Here's the drawing with two shaded views (mm, measured from the low corner). I have some questions. Coordinates: 2 decimals unless noted, no trailing zeros. Order: outer loops, then holes, each group sorted by start corner. A loop starts at its lowest first (then second) coordinate and runs counter-clockwise, first axis right, second up. Notation, with made-up numbers: (-25.5, 30) -> (24.5, 30) arc R22 ccw to (24.5, 37) -> close; hole circle Ø7 at (14, 53). An arc over 180 degrees is marked (long way). Answer in a Markdown table with one row per item. Add a question column.
1. Imagine slicing it at B-B on x = 63. Write out the boundary of the cut face in (y, z), plus the area to 3 significant figures.
2. Will these pins go through, and if not, where does the flat tip stop? pin 1 (1.5 mm diameter, centred on x = 64.5, z = 1.5, fed in from +Y); pin 2 (1 mm diameter, centred on x = 17, z = 2.5, fed in from -Y).
3. Imagine slicing it at A-A on z = 1.8. Write out the boundary of the cut face in (x, y).
4. If I drill on line 1 along X through (y, z) = (50.5, 1.9); line 2 along Y through (x, z) = (39, 1.3), over which ranges is the centre line in solid material (lowest first)? Write a range as [from, to].
5. Imagine slicing it at C-C on x = 16.05. Write out the boundary of the cut face in (y, z), plus the area to 3 significant figures.
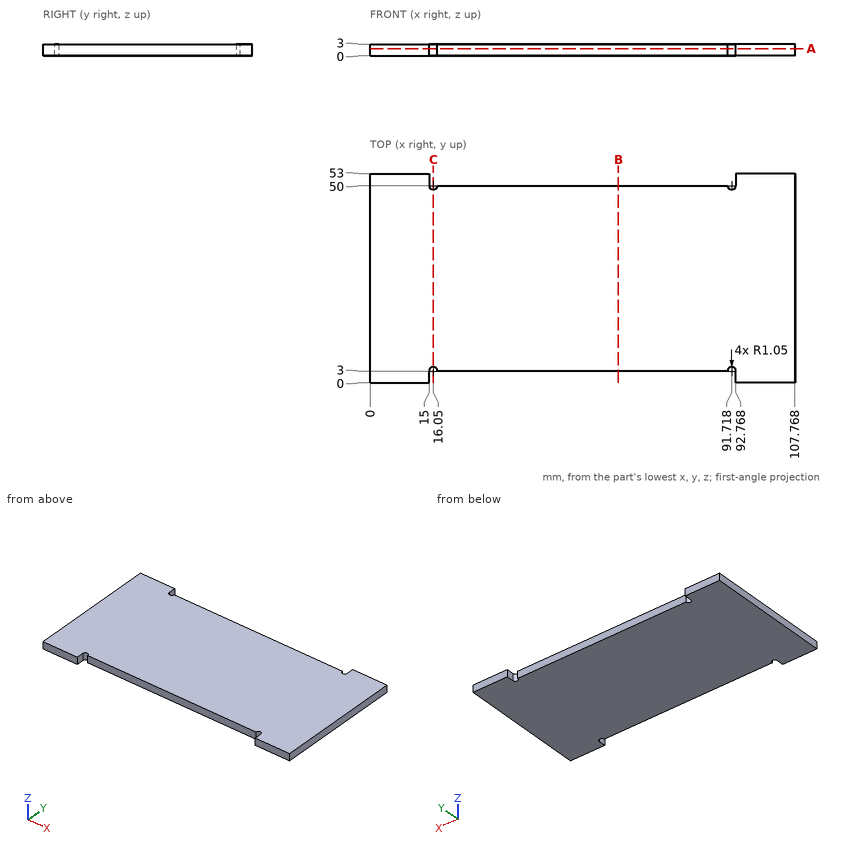
Answers follow:
| question | item | result |
|---|---|---|
| 1 | outline | (3, 0) -> (50, 0) -> (50, 3) -> (3, 3) -> close |
| 1 | area | 141 mm² |
| 2 | pin 1 | stops at y = 50 |
| 2 | pin 2 | stops at y = 3 |
| 3 | outline | (0, 0) -> (15, 0) -> (15, 3) arc R1.05 cw to (17.1, 3) -> (90.67, 3) arc R1.05 cw to (92.77, 3) -> (92.77, 0) -> (107.77, 0) -> (107.77, 53) -> (92.77, 53) -> (92.77, 50) arc R1.05 cw to (90.67, 50) -> (17.1, 50) arc R1.05 cw to (15, 50) -> (15, 53) -> (0, 53) -> close |
| 4 | line 1 | x = [0, 15], [92.77, 107.77] |
| 4 | line 2 | y = [3, 50] |
| 5 | outline | (4.05, 0) -> (48.95, 0) -> (48.95, 3) -> (4.05, 3) -> close |
| 5 | area | 135 mm² |
